Verification items for this drawing (mm, ordinates from the low corner). Round coordinates to 2 decimals unless told otherwise and drop trailing zeros. Write each loop counter-clockwise with the first axis right and the second up, starting at its lowest first coordinate (ties: lowest second). Pieces come first, ordered by that corner, then holes.
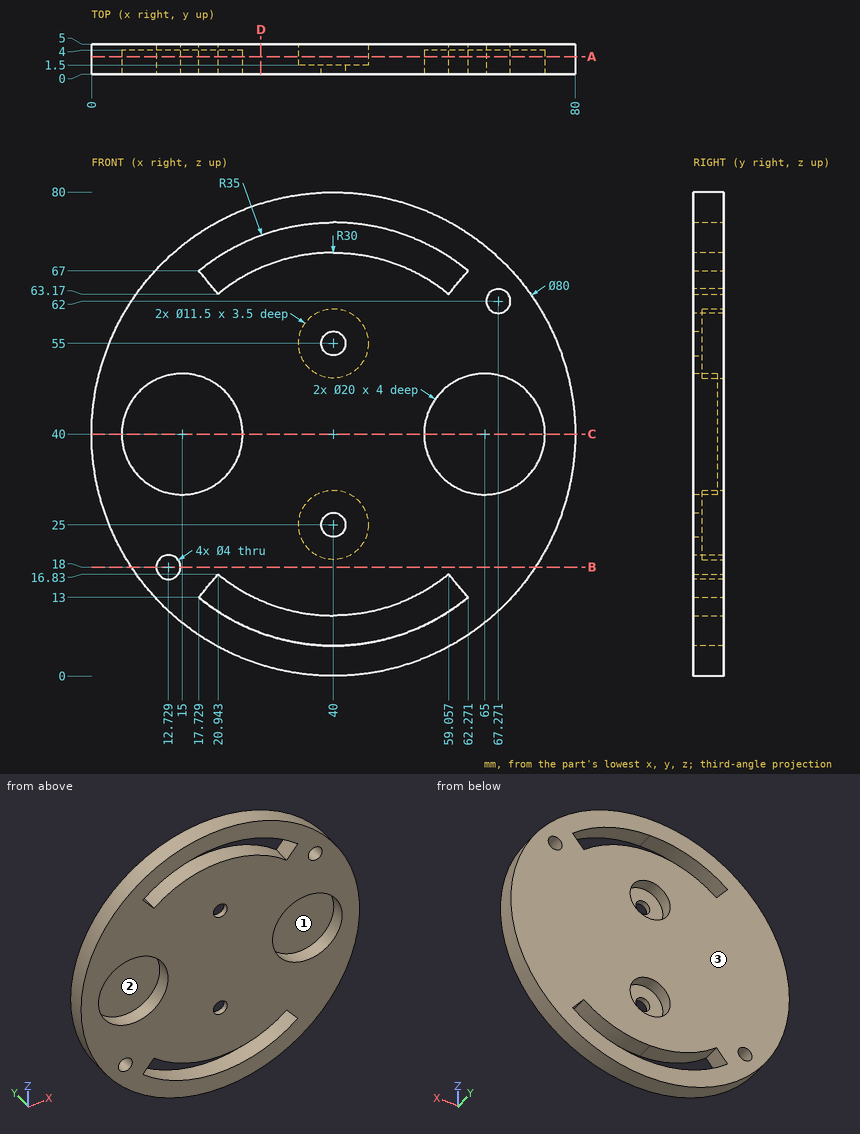
1. Release check for a two-part mould opening along X. For the marked faces 1, 2 and 3 record: +X half, -X half, draft (parallel to the pull), parting line (faces both ways), or undercut.
2. Depth check by flat-ended pin: pin 1 Ø2 at (x, y) = (60, 1) entering from -Z; pin 2 Ø10 at (x, z) = (65, 35.5) entering from -Y; pin 3 Ø3.5 at (x, z) = (40.5, 56) entering from +Y. Enter the tip coordinate at first touch or a pass-through.
3. Section check D-D (x = 28). Record the cut outline in (y, z) (1 decimal), plus the area to 3 significant figures.
4. Section check C-C (z = 40). Record the cut outline in (x, y).
5. Scan lines: line 1 along Z through (x, y) = (40, 2.8); line 2 along Z through (x, y) = (40, 1.15); line 3 along Z through (x, y) = (26, 3.8). Record each from-to range of solid material in increasing order.
6. Section check B-B (z = 18). Record the cut outline in (x, y).
7. Section check A-A (y = 2.9). State how many separate pieces and enclosed holes the cut face has, plus the area to 3 significant figures.
Results below:
1. face 1: undercut
1. face 2: undercut
1. face 3: draft
2. pin 1: stops at z = 4.8
2. pin 2: stops at y = 4
2. pin 3: stops at y = 1.5
3. outline: (0, 1.8) - (5, 1.8) - (5, 7.1) - (0, 7.1) - close; (0, 12.5) - (5, 12.5) - (5, 67.5) - (0, 67.5) - close; (0, 72.9) - (5, 72.9) - (5, 78.2) - (0, 78.2) - close
3. area: 328 mm2
4. outline: (0, 0) - (5, 0) - (5, 4) - (25, 4) - (25, 0) - (55, 0) - (55, 4) - (75, 4) - (75, 0) - (80, 0) - (80, 5) - (0, 5) - close
5. line 1: z = 0 to 5, 10 to 19.25, 30.75 to 49.25, 60.75 to 70, 75 to 80
5. line 2: z = 0 to 5, 10 to 23, 27 to 53, 57 to 70, 75 to 80
5. line 3: z = 2.53 to 7.92, 13.47 to 66.53, 72.08 to 77.47
6. outline: (6.59, 0) - (10.73, 0) - (10.73, 5) - (6.59, 5) - close; (14.73, 0) - (73.41, 0) - (73.41, 5) - (14.73, 5) - close
7. separate pieces: 1
7. enclosed holes: 8
7. area: 3,720 mm2
